Could you check a few things on this model? Use its own coordinates, in mm. Face numbers are marked on the shaded views. A direction names the side the tool comes from. Coordinates: 2 decimals unless noted, no trailing zeros. Loops run counter-clockwise (first coordinate to the right, second up) from the corner with the lowest first, then second, coordinate; pieces in that order, holes last.
1) Imagine slicing it at B-B on z = 2.8. Please give me the cut outline in (x, y).
2) Thinking about a two-plate mould opening in Y: for the marked faces 1, 2, 3 and 4, which applies, released by +Y, released by -Y, zero draft, split by the parting line, or undercut?
3) Imagine slicing it at C-C on x = 4.25. Please give me the cut outline in (y, z).
4) If I drill on line 1 along Y through (x, z) = (-2.5, 2.7); line 2 along Z through (x, y) = (0, 4.25); line 3 along X through (y, z) = (-2.5, 1), over which ranges is the centre line in solid material (lowest first)?
5) For the marked faces 5, 6 and 7, which set-ups out of +Z, -Z, +X, -X, +Y, -Y let a thin tool reach every point of the face, with its end or its side?
6) Will these pins go through, and if not, where does the flat tip stop? P1, Ø3, axis at x = -3.78, y = -3.78, coming from the +Z side; P2, Ø0.6, axis at y = 3.5, z = 1, coming from the +X side; P3, Ø6.5, axis at x = 2.5, y = 2, coming from the -Z side.
7) Imagine slicing it at D-D on z = 1.8. Please give me the cut outline in (x, y), plus the area to 3 significant figures.
8) Imagine slicing it at A-A on y = -0.5. Please give me the cut outline in (x, z), plus the area to 3 significant figures.
```python
from build123d import *

# Parameters (mm, degrees)
F0_R     = 1.75
F1_DEPTH = 3
F2_DEPTH = 0.5
F3_SIZE  = 0.5
F4_SIZE  = 0.5


with BuildPart() as f1:
    # F0 (on Top) → F1 (new body)
    with BuildSketch(Plane.XY):
        Polygon((6.219204, 1.219204), (1.219204, 1.219204), (1.219204, 6.219204), (-1.780796, 6.219204), (-1.780796, -1.780796), (6.219204, -1.780796), align=None)
        with BuildLine():
            Line((-1.780796, -1.780796), (-1.780796, 6.219204))
            Line((-1.780796, 6.219204), (-6.419294, -2.353096))
            ThreePointArc((-6.419294, -2.353096), (-5.902116, -5.902116), (-2.353096, -6.419294))
            Line((-2.353096, -6.419294), (6.219204, -1.780796))
            Line((6.219204, -1.780796), (-1.780796, -1.780796))
        make_face()
        with Locations((-3.780796, -3.780796)):
            Circle(F0_R, mode=Mode.SUBTRACT)
    extrude(amount=F1_DEPTH)

    # F0 (on Top) → F2 (cut)
    with BuildSketch(Plane.XY):
        Polygon((6.219204, 1.219204), (1.219204, 1.219204), (1.219204, 6.219204), (-1.780796, 6.219204), (-1.780796, -1.780796), (6.219204, -1.780796), align=None)
    extrude(amount=F2_DEPTH, mode=Mode.SUBTRACT)

    # F3
    f3_edges = [f1.edges().sort_by_distance(p)[0] for p in [
        (1.933054, -4.100045, 3),
        (-5.902116, -5.902116, 3),
        (-4.100045, 1.933054, 3),
    ]]
    chamfer(f3_edges, length=F3_SIZE)

    # F4
    f4_edges = [f1.edges().sort_by_distance(p)[0] for p in [
        (6.219204, 0.003457, 3),
        (3.719204, 1.219204, 3),
        (1.219204, 3.719204, 3),
        (0.003457, 6.219204, 3),
    ]]
    chamfer(f4_edges, length=F4_SIZE)


solid = f1.part
```
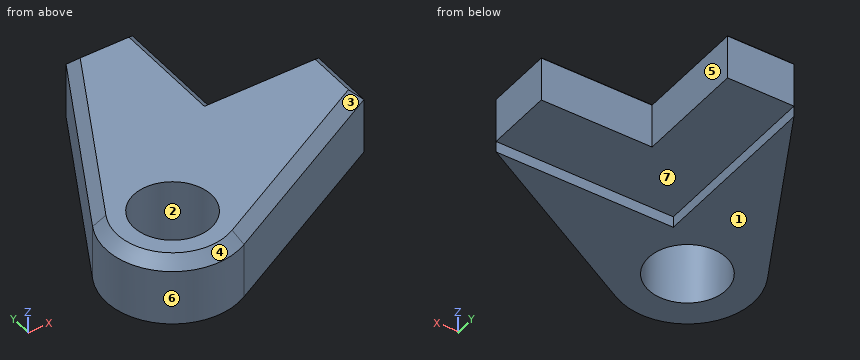
Filled in:
1. outline: (-6.16, -2.5) arc R2.7 ccw to (-2.5, -6.16) - (5.92, -1.6) - (5.92, 0.92) - (0.92, 0.92) - (0.92, 5.92) - (-1.6, 5.92) - close; hole circle Ø3.5 at (-3.78, -3.78)
2. face 1: zero draft
2. face 2: undercut
2. face 3: released by -Y
2. face 4: split by the parting line
3. outline: (-2.85, 0) - (-1.78, 0) - (-1.78, 0.5) - (1.22, 0.5) - (1.22, 2.5) - (0.72, 3) - (-2.28, 3) - (-2.85, 2.5) - close
4. line 1: y = -6.27 to -4.97, -2.59 to 4.47
4. line 2: z = 0.5 to 3
4. line 3: x = -6.49 to -4.97, -2.59 to 4.89
5. face 5: +Z, -Z, +X, +Y
5. face 6: +Z, -Z
5. face 7: -Z, +X, +Y
6. P1: passes through
6. P2: stops at x = 1.22
6. P3: stops at z = 0.5
7. outline: (-6.42, -2.35) arc R3 ccw to (-2.35, -6.42) - (6.22, -1.78) - (6.22, 1.22) - (1.22, 1.22) - (1.22, 6.22) - (-1.78, 6.22) - close; hole circle Ø3.5 at (-3.78, -3.78)
7. area: 86.2 mm2
8. outline: (-5.42, 0) - (-1.78, 0) - (-1.78, 0.5) - (6.22, 0.5) - (6.22, 2.5) - (5.72, 3) - (-4.85, 3) - (-5.42, 2.5) - close
8. area: 30.6 mm2
